Geometry check sheet. Reference: drawing and pictorial views, mm from the part's lowest x, y, z. A direction names the side the tool comes from. Give positions to 0.01 mm unless a question says otherwise; leave off trailing zeros. Order: outer loops, then holes, each group sorted by start corner. A loop starts at its lowest first (then second) coordinate and runs counter-clockwise, first axis right, second up.
Item 1: Gauge pin test, flat ends, axial feed: P1, Ø5, axis at x = 18.5, y = 6, coming from the +Z side; P2, Ø2, axis at y = 7, z = 16.5, coming from the +X side; P3, Ø4, axis at x = 13, y = 9.5, coming from the -Z side. Record the tip position at first contact, or that the pin passes through.
Item 2: Sectioned sample at B-B on z = 22.5. Record the boundary of the cut face in (x, y).
Item 3: Sectioned sample at A-A on x = 18. Record the boundary of the cut face in (y, z).
Item 4: Release check for a two-part mould opening along Z. For the marked faces 5, 6 and 7 record: released by +Z, released by -Z, zero draft, split by the parting line, or undercut.
Item 5: Sectioned sample at D-D on x = 7.5. Record the boundary of the cut face in (y, z), and give its area (3 significant figures).
Item 6: Sectioned sample at C-C on y = 9.75. Record the boundary of the cut face in (x, z).
Item 7: Access from +Z, -Z, +X, -X, +Y, -Y to the whole of each face (thin tool, end or side, straight path). Record for the marked faces 1, 2, 3 and 4.
Item 8: Material ranges on line 1 along Y through (x, z) = (22.5, 39); line 2 along X through (y, z) = (10.5, 22); line 3 along X through (y, z) = (2.5, 29), recorded low to high.
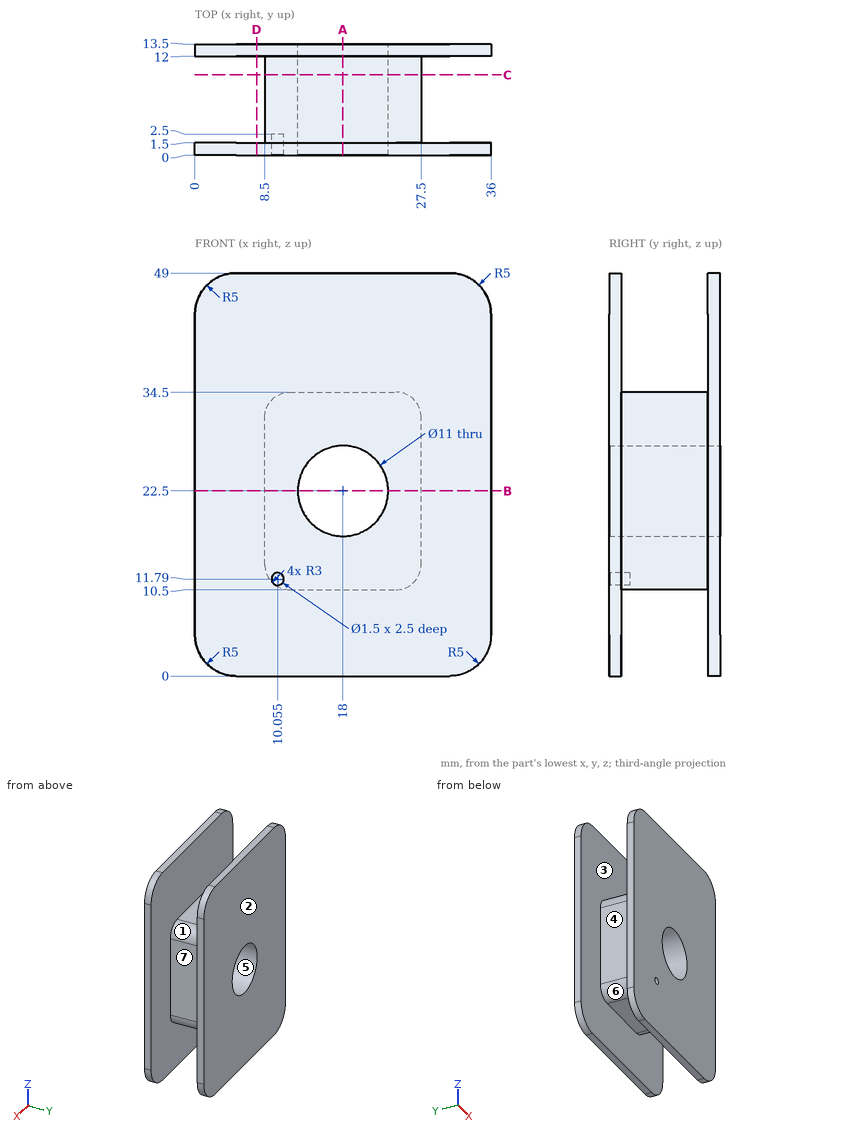
Report:
1. P1: stops at z = 34.5
1. P2: stops at x = 27.5
1. P3: stops at z = 10.5
2. outline: (0, 0) - (12.5, 0) - (12.5, 13.5) - (0, 13.5) - (0, 12) - (8.5, 12) - (8.5, 1.5) - (0, 1.5) - close; (23.5, 0) - (36, 0) - (36, 1.5) - (27.5, 1.5) - (27.5, 12) - (36, 12) - (36, 13.5) - (23.5, 13.5) - close
3. outline: (0, 0) - (1.5, 0) - (1.5, 10.5) - (12, 10.5) - (12, 0) - (13.5, 0) - (13.5, 17) - (0, 17) - close; (0, 28) - (13.5, 28) - (13.5, 49) - (12, 49) - (12, 34.5) - (1.5, 34.5) - (1.5, 49) - (0, 49) - close
4. face 5: undercut
4. face 6: released by -Z
4. face 7: zero draft
5. outline: (0, 0) - (1.5, 0) - (1.5, 49) - (0, 49) - close; (12, 0) - (13.5, 0) - (13.5, 49) - (12, 49) - close
5. area: 147 mm2
6. outline: (8.5, 13.5) arc R3 ccw to (11.5, 10.5) - (24.5, 10.5) arc R3 ccw to (27.5, 13.5) - (27.5, 31.5) arc R3 ccw to (24.5, 34.5) - (11.5, 34.5) arc R3 ccw to (8.5, 31.5) - close; hole circle Ø11 at (18, 22.5)
7. face 1: +Z, +X
7. face 2: +Z, -Z, +X, -X, +Y
7. face 3: none
7. face 4: +Z, -Z, -X
8. line 1: y = 0 to 1.5, 12 to 13.5
8. line 2: x = 8.5 to 12.52, 23.48 to 27.5
8. line 3: x = 8.5 to 27.5
